from build123d import *

# Parameters (mm, degrees)
EXTRUDE_1_DEPTH     = 100
EXTRUDE_2_DEPTH     = 100
EXTRUDE_3_DEPTH     = 100
EXTRUDE_START       = -100
EXTRUDE_4_DEPTH     = 100
CUT_EXTRUDE_1_DEPTH = 1221.655561574
EXTRUDE_1_2_DEPTH   = 100
CUT_EXTRUDE_2_DEPTH = 1226.38987213


# Read off the part's stored shape, not the designer's step: 拉伸-薄壁4
with BuildPart() as part:
    # 草图1 → Extrude 1 (new body)
    with BuildSketch(Plane.XY):
        Polygon((-600, 0), (-400, 346.410161514), (-200, 0), (-400, -346.410161514), align=None)
        Polygon((-588.452994616, 0), (-400, 326.410161514), (-211.547005384, 0), (-400, -326.410161514), align=None, mode=Mode.SUBTRACT)
    extrude(amount=-EXTRUDE_1_DEPTH)

    # 草图1<4> → 拉伸-薄壁2 (add)
    with BuildSketch(Plane.XY):
        Polygon((400, -346.410161514), (200, -692.820323028), (-200, -692.820323028), (-400, -346.410161514), (-200, 0), (0, 0), (200, 0), align=None)
        Polygon((388.452994616, -346.410161514), (194.226497308, -682.820323028), (-194.226497308, -682.820323028), (-388.452994616, -346.410161514), (-194.226497308, -10), (0, -10), (194.226497308, -10), align=None, mode=Mode.SUBTRACT)
    extrude(amount=-EXTRUDE_2_DEPTH)

    # 草图1<5> → 拉伸-薄壁3 (add)
    with BuildSketch(Plane.XY):
        Polygon((400, -346.410161514), (200, 0), (400, 346.410161514), (600, 0), align=None)
        Polygon((400, -326.410161514), (211.547005384, 0), (400, 326.410161514), (588.452994616, 0), align=None, mode=Mode.SUBTRACT)
    extrude(amount=-EXTRUDE_3_DEPTH)

    # 拉伸-薄壁4 outline → 拉伸-薄壁4 (add)
    with BuildSketch(Plane.XY.offset(EXTRUDE_START)):
        Polygon((200, 692.820323028), (-200, 692.820323028), (-400, 346.410161514), (-200, 0), (200, 0), (400, 346.410161514), align=None)
        Polygon((-194.226497308, 10), (-388.452994616, 346.410161514), (-194.226497308, 682.820323028), (194.226497308, 682.820323028), (388.452994616, 346.410161514), (194.226497308, 10), align=None, mode=Mode.SUBTRACT)
    extrude(amount=EXTRUDE_4_DEPTH)

    # 草图4 → 切除-拉伸1 (cut, through all)
    with BuildSketch(Plane(origin=(-400, 0, 0), x_dir=(0, 0, -1), z_dir=(1, 0, 0))):
        Polygon((50, 0), (0, -326.410161514), (0, 0), (0, 326.410161514), align=None)
    cut_extrude_1 = extrude(amount=-CUT_EXTRUDE_1_DEPTH, mode=Mode.SUBTRACT)

    # 镜向1: 切除-拉伸1 across plane
    add(cut_extrude_1.mirror(Plane(origin=(0, 0, 0), x_dir=(0, 0, 1), z_dir=(1, 0, 0))), mode=Mode.SUBTRACT)

    # 草图2 → Extrude 1 2 (add)
    with BuildSketch(Plane.XY):
        Polygon((388.452994616, 346.410161514), (400, 326.410161514), (405.773502692, 336.410161514), (200, 692.820323028), (-200, 692.820323028), (-405.773502692, 336.410161514), (-400, 326.410161514), (-388.452994616, 346.410161514), (-194.226497308, 682.820323028), (194.226497308, 682.820323028), align=None)
        Polygon((-400, -326.410161514), (-388.452994616, -346.410161514), (-194.226497308, -10), (194.226497308, -10), (388.452994616, -346.410161514), (400, -326.410161514), (211.547005384, 0), (400, 326.410161514), (388.452994616, 346.410161514), (194.226497308, 10), (-194.226497308, 10), (-388.452994616, 346.410161514), (-400, 326.410161514), (-211.547005384, 0), align=None)
        Polygon((405.773502692, -336.410161514), (400, -326.410161514), (388.452994616, -346.410161514), (194.226497308, -682.820323028), (-194.226497308, -682.820323028), (-388.452994616, -346.410161514), (-400, -326.410161514), (-405.773502692, -336.410161514), (-200, -692.820323028), (200, -692.820323028), align=None)
    extrude(amount=EXTRUDE_1_2_DEPTH)

    # 草图6 → 切除-拉伸2 (cut, through all)
    with BuildSketch(Plane.ZY.offset(405.773502692)):
        Polygon((100, 692.820323028), (100, 336.410161514), (0, 336.410161514), align=None)
        Polygon((100, 0), (0, 336.410161514), (100, 336.410161514), align=None)
        Polygon((100, 0), (100, -336.410161514), (0, -336.410161514), align=None)
        Polygon((100, -692.820323028), (0, -336.410161514), (100, -336.410161514), align=None)
        Polygon((50, -692.820323028), (100, -692.820323028), (50, -514.615242271), align=None)
        Polygon((50, -514.615242271), (0, -336.410161514), (50, -692.820323028), align=None)
        Polygon((50, -514.615242271), (50, -336.410161514), (0, -336.410161514), align=None)
        Polygon((50, 514.615242271), (0, 336.410161514), (50, 336.410161514), align=None)
        Polygon((50, 692.820323028), (0, 336.410161514), (50, 514.615242271), align=None)
        Polygon((50, 514.615242271), (100, 692.820323028), (50, 692.820323028), align=None)
    extrude(amount=-CUT_EXTRUDE_2_DEPTH, mode=Mode.SUBTRACT)


solid = part.part
Could you check a few things on this model? Use its own coordinates, in mm. A direction names the side the tool comes from. Round coordinates to 2 decimals unless told otherwise and drop trailing zeros. Write each loop counter-clockwise with the first axis right and the second up, starting at its lowest first coordinate (ties: lowest second). Pieces come first, ordered by that corner, then holes. Notation, with made-up numbers: (39, 16) - (92, 16) arc R25 cw to (92, 33) - close; hole circle Ø3 at (78, -34). An arc over 180 degrees is marked (long way). Put each result on its own line as item: value. Start each with the question number.
(1) I need wall thicknesses on probe 1 along Y at (x, z) = (163.5, 43.5); probe 2 along Y at (x, z) = (329, -7.5); probe 3 along X at (y, z) = (211, -45.5). Which ranges of each line are inside material? Lowest first, please.
(2) Will these pins go through, and if not, where does the flat tip stop? pin 1 (2 mm diameter, centred on x = 6, z = 64.5, fed in from -Y); pin 2 (5 mm diameter, centred on x = 404.5, y = 329.5, fed in from +Z); pin 3 (11 mm diameter, centred on x = -403.5, y = -331.5, fed in from +Z).
(3) Thinking about a two-plate mould opening in Y: for faces 1 (the flat face through (-358.356, -418.54, -42.717)), 2 (the flat face through (-292.7, -180.56, -24.76)), 3 (the flat face through (3, 692.82, -26)), which applies, released by +Y, released by -Y, zero draft, split by the parting line, or undercut?
(4) For faces 4 (the flat face through (352.756, -428.24, -42.717)), 5 (the flat face through (-31.951, -685.389, 48.957)), 6 (the flat face through (-289.98, 175.85, -24.76)), 7 (the flat face through (-499.533, 163.967, -24.883)), 8 (the flat face through (358.356, 418.54, -42.717)), which set-ups out of +Z, -Z, +X, -X, +Y, -Y let a thin tool reach every point of the face, with its end or its side?
(5) I want a section at D-D, the plane x = 436.5. Please give me the cut outline in (y, z), plus the area to 3 significant figures.
(6) I want a section at B-B, the plane y = 135. Please give me the cut outline in (x, z).
(7) I want a section at A-A, the plane x = -73. Please give me the cut outline in (y, z), plus the area to 3 significant figures.
(8) I want a section at C-C, the plane y = 423. Please give me the cut outline in (x, z).
Here are the results:
1. probe 1: y = -692.82 to -682.82, -10 to 10, 682.82 to 692.82
1. probe 2: y = -469.39 to -449.39, -243.43 to -203.43, 203.43 to 243.43, 449.39 to 469.39
1. probe 3: x = -478.18 to -466.63, -333.37 to -310.27, 310.27 to 333.37, 466.63 to 478.18
2. pin 1: stops at y = -10
2. pin 2: stops at z = 1.92
2. pin 3: stops at z = 2.8
3. face 1: released by -Y
3. face 2: undercut
3. face 3: released by +Y
4. face 4: +Z, -Z, +X, -Y
4. face 5: +Z, +X, -X
4. face 6: +Z, -Z
4. face 7: +Z, -X
4. face 8: +Z, -Z, +X, +Y
5. outline: (-283.19, -100) - (-263.19, -100) - (-263.19, -9.68) - (-283.19, -6.62) - close; (263.19, -100) - (283.19, -100) - (283.19, -6.62) - (263.19, -9.68) - close
5. area: 3,670 mm^2
6. outline: (-522.06, -100) - (-510.51, -100) - (-510.51, -29.32) - (-522.06, -29.32) - close; (-289.49, -100) - (-266.4, -100) - (-266.4, 59.87) - (-289.49, 59.87) - close; (266.4, -100) - (289.49, -100) - (289.49, 59.87) - (266.4, 59.87) - close; (510.51, -100) - (522.06, -100) - (522.06, -29.32) - (510.51, -29.32) - close
7. outline: (-692.82, -100) - (-682.82, -100) - (-682.82, 48.6) - (-692.82, 50) - close; (-10, -100) - (10, -100) - (10, 97.03) - (0, 100) - (-10, 97.03) - close; (682.82, -100) - (692.82, -100) - (692.82, 50) - (682.82, 48.6) - close
7. area: 6,960 mm^2
8. outline: (-355.78, -100) - (-344.23, -100) - (-344.23, 12.15) - (-355.78, 12.15) - close; (344.23, -100) - (355.78, -100) - (355.78, 12.15) - (344.23, 12.15) - close
